Read the model definition and answer for the solid it produces. Units are mm, in the model's axes. Give positions to 0.01 mm unless a question says otherwise; leave off trailing zeros. Write each loop counter-clockwise with the first axis right and the second up, starting at its lowest first coordinate (ties: lowest second). Pieces come first, ordered by that corner, then holes. Notation, with made-up numbers: M 59,-6.5 L 83,-6.5 A30 ccw 83,15.5 Z; hole C -24.75,74 d9. An arc over 180 degrees is marked long. Put each result on its own line as item: value.
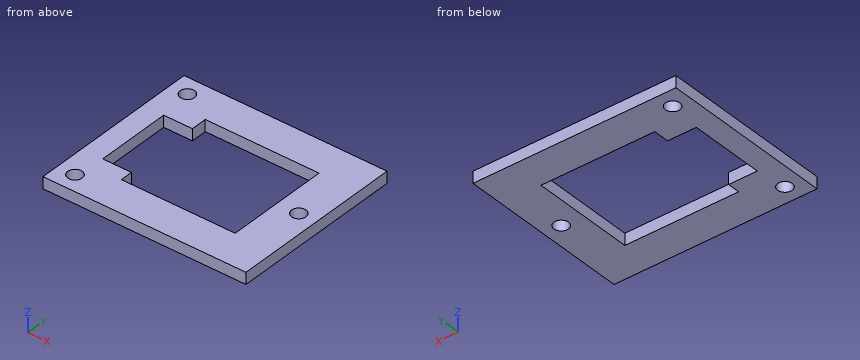
from build123d import *

# Parameters (mm, degrees)
F0_W     = 35
F0_H     = 30
F0_R     = 1.25
F1_DEPTH = 2


with BuildPart() as f1:
    # F0 (on Top) → F1 (new body)
    with BuildSketch(Plane.XY):
        Rectangle(F0_W, F0_H)
        with Locations((-14.45, -11.95)):
            Circle(F0_R, mode=Mode.SUBTRACT)
        Polygon((-8.916158, 8.917894), (8.916158, 8.917894), (10.707928, 8.917894), (10.707925, -8.917894), (8.916158, -8.917894), (-8.916158, -8.917894), (-8.916158, -6.781416), (-13.864904, -6.781416), (-13.864904, 6.187579), (-8.916158, 6.187579), align=None, mode=Mode.SUBTRACT)
        with Locations((-14.45, 11.95)):
            Circle(F0_R, mode=Mode.SUBTRACT)
        with Locations((14.45, 0)):
            Circle(F0_R, mode=Mode.SUBTRACT)
    extrude(amount=F1_DEPTH)


solid = f1.part
(1) Straight lines are drawn through the part: line 1 along Y through (x, z) = (-14.45, 0.7); line 2 along Y through (x, z) = (2.5, 0.7); line 3 along Y through (x, z) = (-15, 1.7). For each, find the intervals that lie inside material, in ascending order. Write a range as from..to.
Result:
line 1: y = -15..-13.2, -10.7..10.7, 13.2..15
line 2: y = -15..-8.92, 8.92..15
line 3: y = -15..-13.07, -10.83..10.83, 13.07..15
(2) Section C-C on z = 1 is taken. Determine the outline of the cut face in (x, y).
Result:
outline: M -17.5,-15 L 17.5,-15 L 17.5,15 L -17.5,15 Z; hole C -14.45,-11.95 d2.5; hole C -14.45,11.95 d2.5; hole M -13.86,-6.78 L -8.92,-6.78 L -8.92,-8.92 L 10.71,-8.92 L 10.71,8.92 L -8.92,8.92 L -8.92,6.19 L -13.86,6.19 Z; hole C 14.45,0 d2.5
(3) Section B-B on y = -11.95 is taken. Determine the outline of the cut face in (x, z).
Result:
outline: M -17.5,0 L -15.7,0 L -15.7,2 L -17.5,2 Z; M -13.2,0 L 17.5,0 L 17.5,2 L -13.2,2 Z
(4) Section A-A on x = -9.5 is taken. Determine the outline of the cut face in (y, z), and give its area (3 significant figures).
Result:
outline: M -15,0 L -6.78,0 L -6.78,2 L -15,2 Z; M 6.19,0 L 15,0 L 15,2 L 6.19,2 Z
area: 34.1 mm²
(5) Given pin 1 Ø2 at (x, y) = (-14.45, 11.95) entering from -Z, flat-ended and moving along its own axis, determine where the tip first touches the part or whether it passes through.
Result:
pin 1: passes through
(6) Section D-D on y = 0 is taken. Determine the outline of the cut face in (x, z), and give its area (3 significant figures).
Result:
outline: M -17.5,0 L -13.86,0 L -13.86,2 L -17.5,2 Z; M 10.71,0 L 13.2,0 L 13.2,2 L 10.71,2 Z; M 15.7,0 L 17.5,0 L 17.5,2 L 15.7,2 Z
area: 15.9 mm²
